```python
from build123d import *

# Parameters (mm, degrees)
SKETCH002_W     = 4
SKETCH002_H     = 13
SKETCH002_R     = 1.5
PAD002_DEPTH    = 10
SKETCH003_W     = 12.732194
SKETCH003_H     = 9.787396
POCKET_DEPTH    = 5
SKETCH004_R     = 1.5
POCKET001_DEPTH = 5


with BuildPart() as part:
    # Sketch002 → Pad002 (new body)
    with BuildSketch(Plane.XY):
        with Locations((-10.268592, 10.465797)):
            Rectangle(SKETCH002_W, SKETCH002_H)
        with Locations((-10.253053, 11.743256)):
            Circle(SKETCH002_R, mode=Mode.SUBTRACT)
    extrude(amount=-PAD002_DEPTH)

    # Sketch003 (on Face2 of Pad002) → Pocket (cut)
    with BuildSketch(Plane.YZ.offset(-8.268592)):
        with Locations((10.199147, -5.293698)):
            Rectangle(SKETCH003_W, SKETCH003_H)
    extrude(amount=-POCKET_DEPTH, mode=Mode.SUBTRACT)

    # Sketch004 (on Face6 of Pocket) → Pocket001 (cut)
    with BuildSketch(Plane(origin=(0, 16.965797, 0), x_dir=(-1, 0, 0), z_dir=(0, 1, 0))):
        with Locations((10.62654, -4.306276)):
            Circle(SKETCH004_R)
    extrude(amount=-POCKET001_DEPTH, mode=Mode.SUBTRACT)


solid = part.part
```
Geometry: final body of the model. Coordinates: model frame, mm. A direction names the side the tool comes from. Give positions to 0.01 mm unless a question says otherwise; leave off trailing zeros. Loops run counter-clockwise (first coordinate to the right, second up) from the corner with the lowest first, then second, coordinate; pieces in that order, holes last. Notation, with made-up numbers: (79, 18) -> (118, 18) arc R19 ccw to (118, 40) -> close; hole circle Ø8 at (54.5, 66). An arc over 180 degrees is marked (long way). Return JSON: item names as keys, results as strings.
Item 1: Section B-B, the plane y = 12.75. Output: boundary loops of the cut face in (x, z), plus the area to 3 significant figures.
Filled in:
{"outline": "(-12.27, -0.4) -> (-11.37, -0.4) -> (-11.37, 0) -> (-12.27, 0) -> close; (-9.14, -0.4) -> (-8.27, -0.4) -> (-8.27, 0) -> (-9.14, 0) -> close", "area": "0.710 mm^2"}
Item 2: Section A-A, the plane x = -9.35. Output: boundary loops of the cut face in (y, z), plus the area to 3 significant figures.
Filled in:
{"outline": "(3.97, -0.4) -> (10.55, -0.4) -> (10.55, 0) -> (3.97, 0) -> close; (12.94, -0.4) -> (16.57, -0.4) -> (16.57, -3.52) -> (16.97, -3.52) -> (16.97, 0) -> (12.94, 0) -> close; (16.57, -10) -> (16.97, -10) -> (16.97, -5.09) -> (16.57, -5.09) -> close", "area": "7.46 mm^2"}
Item 3: Section D-D, the plane z = -7. Output: boundary loops of the cut face in (x, y), plus the area to 3 significant figures.
Filled in:
{"outline": "(-12.27, 16.57) -> (-8.27, 16.57) -> (-8.27, 16.97) -> (-12.27, 16.97) -> close", "area": "1.60 mm^2"}
Item 4: Pin query (flat end, axial travel): P1, Ø2, axis at x = -9.5, y = 13.5, coming from the -Z side; P2, Ø5, axis at y = 9.5, z = -4.5, coming from the -X side. Return the tip coordinate at first contact, or that it passes through.
Filled in:
{"P1": "z = -0.4", "P2": "through"}
Item 5: Mould query, pull axis X, two halves, no side actions, for faces 3 (the flat face through (-8.269, 13.3, -0.2)), 4 (the cylindrical face through (-11.75, 11.81, -0.2)), 5 (the flat face through (-10, 9, 0)), 6 (the cylindrical face through (-9.436, 16.768, -5.219)). Classes: released by +X, released by -X, zero draft, split by the parting line, or undercut.
Filled in:
{"face 3": "released by +X", "face 4": "undercut", "face 5": "zero draft", "face 6": "undercut"}
Item 6: Access query for faces 1 (the flat face through (-12.269, 13.3, -0.2)), 2 (the flat face through (-10, 10, -0.4)). Directions: +Z, -Z, +X, -X, +Y, -Y. A direction counts if a zero-diameter tool reaches every point of the face in a straight line with its end or side. Return the directions, or none.
Filled in:
{"face 1": "+Z, -Z, -X, +Y, -Y", "face 2": "-Z, +X, -X, -Y"}
Item 7: Section C-C, the plane x = -11.9. Output: boundary loops of the cut face in (y, z), plus the area to 3 significant figures.
Filled in:
{"outline": "(3.97, -0.4) -> (16.57, -0.4) -> (16.57, -3.51) -> (16.97, -3.51) -> (16.97, 0) -> (3.97, 0) -> close; (16.57, -10) -> (16.97, -10) -> (16.97, -5.1) -> (16.57, -5.1) -> close", "area": "8.41 mm^2"}
Item 8: Line query: line 1 (Z direction, x = -8.9, y = 8.5); line 2 (Y direction, x = -8.75, z = -4). Output: solid intervals per line, ascending.
Filled in:
{"line 1": "-0.4 to 0", "line 2": "16.57 to 16.97"}
